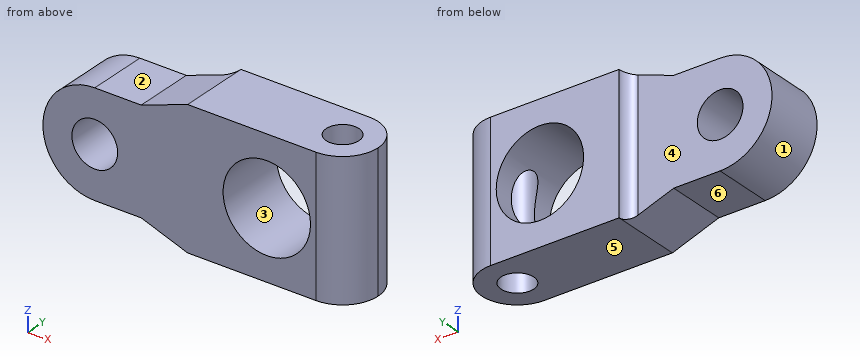
Autodesk Inventor part; units mm, degrees
ref_plane "YZ Plane" through (0, 0, 0) normal (1, 0, 0) x (0, 1, 0)
ref_plane "XZ Plane" through (0, 0, 0) normal (0, 1, 0) x (-1, 0, 0)
ref_plane "XY Plane" through (0, 0, 0) normal (0, 0, 1) x (1, 0, 0)
sketch "Skizze1" plane through (0, 0, 0) normal (0, 1, 0) x (-1, 0, 0)
  line L0 (0, 12.5) -> (0, -12.5)
  line L1 (0, -12.5) -> (30, -12.5)
  arc A0 (47, -9.5) -> (47, 9.5) centre (47, 0) ccw
  line L2 (47, 9.5) -> (38.5, 9.5)
  line L3 (38.5, 9.5) -> (30, 12.5)
  line L4 (30, 12.5) -> (0, 12.5)
  line L5 (0, 0) -> (47, 0) construction
  line L6 (30, -12.5) -> (38.5, -9.5)
  line L7 (38.5, -9.5) -> (47, -9.5)
  line L8 (30, 12.5) -> (30, -12.5)
  point P0 (56.5, 0)
  dimension "d0" = 90
  dimension "d1" = 25
  dimension "d2" = 30
  dimension "d3" = 47
  dimension "d5" = 8.5
  dimension "d6" = 18
  dimension "d9" = 30
extrude "Extrusion2" add sketch "Skizze1" along normal blind 13 contours L4 L8 L1 L0
extrude "Extrusion3" add sketch "Skizze1" along normal blind 11 contours L3 L2 A0 L7 L6 L8
fillet "Rundung1" radius 2 1 edges at (-30, 11, 0)
fillet "Rundung2" radius 6.5 2 edges at (0, 0, 0) (0, 13, 0)
sketch "Skizze2" plane through (-30, 0, -12.5) normal (0, 0, -1) x (-1, 0, 0)
  arc A0 (-23.5, 13) -> (-23.5, 0) centre (-23.5, 6.5) ccw
  point P0 (-30, 0)
hole "Bohrung1" at (-6.5, 6.5, -12.5) direction (0, 0, 1) diameter 6 depth 25
sketch "Skizze3" plane through (0, 11, 0) normal (0, 1, 0) x (1, 0, 0)
  arc A0 (-47, 9.5) -> (-47, -9.5) centre (-47, 0) ccw
  point P0 (0, 0)
hole "Bohrung2" at (-47, 11, 0) direction (0, -1, 0) diameter 8.376 depth 11
sketch "Sketch4" plane through (0, 0, 0) normal (0, -1, 0) x (1, 0, 0)
  circle A0 centre (-15.5, 0) radius 8
  line L0 (-6.5, 12.5) -> (-6.5, -12.5)
  point P0 (0, 0)
  dimension "d30" = 16
  dimension "d33" = 9
extrude "Extrusion4" cut sketch "Sketch4" against normal up to surface (13 mm away)
properties part number "2012"
Design review of the part built by this model. Coordinates are the model's own, in mm. Face numbers are marked on the shaded views. A direction names the side the tool comes from. Round coordinates to 2 decimals unless told otherwise and drop trailing zeros. Order: outer loops, then holes, each group sorted by start corner. A loop starts at its lowest first (then second) coordinate and runs counter-clockwise, first axis right, second up.
1) Consider section A-A (y = 4.75). State the section outline as (x, z) points, plus the area to 3 significant figures.
The answers:
outline: (-47, -9.5) - (-38.5, -9.5) - (-30, -12.5) - (-8.94, -12.5) - (-8.94, -4.57) arc R8 cw (long way) to (-8.94, 4.57) - (-8.94, 12.5) - (-30, 12.5) - (-38.5, 9.5) - (-47, 9.5) arc R9.5 ccw to start; (-4.06, -12.5) - (-0.24, -12.5) - (-0.24, 12.5) - (-4.06, 12.5) - close; hole circle Ø8.38 at (-47, 0)
area: 865 mm2
2) Clearance check with flat-ended pins moving along their axes: pin 1 Ø2 at (y, z) = (6, -7) entering from -X; pin 2 Ø12 at (x, z) = (-47, 3) entering from +Y; pin 3 Ø3 at (y, z) = (3, 2) entering from -X. State where each tip first meets the part, or that it passes through.
The answers:
pin 1: stops at x = -54.37
pin 2: stops at y = 11
pin 3: stops at x = -56.49
3) For L1, parallel to Z at x = -15.5, y = 7.75; L2, parallel to X at y = 6.75, z = 3.75; L3, parallel to Y at x = -6.5, z = 3.75, list the stretches that pass through material, from the lowest coordinate up.
The answers:
L1: z = -12.5 to -8, 8 to 12.5
L2: x = -55.73 to -48.86, -45.14 to -22.57, -3.51 to 0
L3: y = 0 to 3.5, 9.5 to 13
4) Consider section C-C (x = -15.5). State the section outline as (y, z) points.
The answers:
outline: (0, -12.5) - (13, -12.5) - (13, -8) - (0, -8) - close; (0, 8) - (13, 8) - (13, 12.5) - (0, 12.5) - close
5) Consider section B-B (z = 6). Count the separate pieces of the cut face and the enclosed holes in it, plus the area to 3 significant figures.
The answers:
separate pieces: 2
enclosed holes: 1
area: 475 mm2
6) Draft analysis for pull direction Z (two halves, no side actions). For the marked faces 1, 2 and 3, state which applies: released by +Z, released by -Z, zero draft, split by the parting line, or undercut.
The answers:
face 1: split by the parting line
face 2: released by +Z
face 3: undercut
7) Machinability: for the marked faces 4, 5 and 6, which of the approach directions +Z, -Z, +X, -X, +Y, -Y give a long, thin tool a straight path to every point of the face, cutting with its end or side? Answer none if there is none.
The answers:
face 4: +Z, -Z, -X, +Y
face 5: -Z, +X, -X, +Y, -Y
face 6: -Z, -X, +Y, -Y
